For this review, take the finished solid that the model builds, in its own axes (mm). A direction names the side the tool comes from. Give positions to 0.01 mm unless a question says otherwise; leave off trailing zeros. One line per item, written item: value.
```python
from build123d import *

# Parameters (mm, degrees)
ESQUISSE2_R                  = 1
ENL_V_MAT_EXTRU_1_DEPTH      = 0.5
R_P_TITION_CIRCULAIRE1_COUNT = 6
ESQUISSE5_R                  = 0.5
ENL_V_MAT_EXTRU_2_DEPTH      = 0.5


with BuildPart() as part:
    # Esquisse1 → Base-R_volution (revolve)
    with BuildSketch(Plane.XY, mode=Mode.PRIVATE) as base_r_volution_sk:
        Polygon((0, 32.449656843), (0.653785579, 33), (1.307571158, 32.449656843), (2.692428842, 32.449656843), (3.346214421, 33), (4, 32.449656843), (4, 26.537069046), (4.5, 26.537069046), (4.5, 24.475834219), (3.627749385, 23.5), (2, 24.475834219), (0.3, 23.5), (0.5, 24.793358266), (0.5, 26.537069046), (0, 26.537069046), align=None)
    revolve(base_r_volution_sk.sketch.rotate(Axis((0, 0, 0), (1, 0, 0)), 90), axis=Axis((0, 0, 0), (1, 0, 0)))

    # Esquisse2 → Enl_v. mat.-Extru.1 (cut)
    with BuildSketch(Plane.ZY):
        with Locations((0, 29.5)):
            Circle(ESQUISSE2_R)
    enl_v_mat_extru_1 = extrude(amount=-ENL_V_MAT_EXTRU_1_DEPTH, mode=Mode.SUBTRACT)

    # R_p_tition circulaire1: Enl_v. mat.-Extru.1 ×6 about axis
    r_p_tition_circulaire1_axis = Axis((-2.3625, 0, 0), (1, 0, 0))
    for i in range(1, R_P_TITION_CIRCULAIRE1_COUNT):
        add(enl_v_mat_extru_1.rotate(r_p_tition_circulaire1_axis, i * 360 / R_P_TITION_CIRCULAIRE1_COUNT), mode=Mode.SUBTRACT)

    # Esquisse5 → Enl_v. mat.-Extru.2 (cut)
    with BuildSketch(Plane.ZY):
        with Locations((31, 0)):
            Circle(ESQUISSE5_R)
        with Locations((28, 0)):
            Circle(ESQUISSE5_R)
    extrude(amount=-ENL_V_MAT_EXTRU_2_DEPTH, mode=Mode.SUBTRACT)


solid = part.part
```
(1) Wall thickness on line 1 (Y direction, x = 0.2, z = 0); line 2 (X direction, y = -12, z = -23); line 3 (X direction, y = -9.5, z = -28): over which ranges is each line inside the solid? List them lowest first. Write a range as from..to.
Answers below:
line 1: y = -32.62..-30.5, -28.5..-26.54, 26.54..28.5, 30.5..32.62
line 2: x = 0.5..4.5
line 3: x = 0..4
(2) Machinability: for faces 1 (the face through (4.25, -26.31, -3.45)), 2 (the face through (0.25, -15.36, -26.34)), 3 (the face through (4.5, 23.5, 7.7)), which of the approach directions +Z, -Z, +X, -X, +Y, -Y give a long, thin tool a straight path to every point of the face, cutting with its end or side? Answer none if there is none.
Answers below:
face 1: +X
face 2: -X
face 3: +Z, -Z, +X, +Y, -Y
(3) For P1, Ø2.5, axis at y = 14.75, z = -25.55, coming from the +X side; P2, Ø0.6, axis at y = -15, z = -26, coming from the -X side; P3, Ø1.5, axis at x = 4, y = -15, coming from the +Z side, all flat-tipped, find the tip position at first contact; note any pin that passes through.
Answers below:
P1: stops at x = 4
P2: stops at x = 0.5
P3: stops at z = 29.58
